The listing builds one solid part. Answer for the finished solid, in the listing's coordinates (mm). A direction names the side the tool comes from. Round coordinates to 2 decimals unless told otherwise and drop trailing zeros. Write each loop counter-clockwise with the first axis right and the second up, starting at its lowest first coordinate (ties: lowest second). Pieces come first, ordered by that corner, then holes.
Item 1: A tool of negligible diameter and unlimited length cuts with its end or side. For faces 1 (the face through (215.9, 19, 627)), 2 (the face through (-4, -3, -609.6)), from which of +Z, -Z, +X, -X, +Y, -Y can it reach the whole face along a straight path? Write none if from no direction.
Item 2: Find the intervals of material crossed by probe 1 along X at (y, z) = (-6, -203); probe 2 along X at (y, z) = (-6, -50); probe 3 along X at (y, z) = (11.5, 946.5), in increasing order.
Item 3: Find section B-B on z = 1362.5. Give the vertices of the cut face in (x, y).
Item 4: Find section A-A on y = 14. Give the vertices of the cut face in (x, z).
Item 5: Find section C-C on x = -20. Give the vertices of the cut face in (y, z).
Item 6: For a pull along X with two mould halves and no side action, classify faces 3 (the face through (-3, 0, 627)), 4 (the face through (304.8, 10, 593)), 5 (the face through (260, 38.1, 627)) as +X half, -X half, draft (parallel to the pull), parting line (faces both ways), or undercut.
```python
from build123d import *

# Parameters (mm, degrees)
F0_W          = 609.6
F0_H          = 1219.2
F1_DEPTH      = 19.05
F2_W          = 88.9
F2_H          = 38.1
F3_DEPTH      = 1219.2
F4_DEPTH      = 2438.4
F4_DEPTH_BACK = 1219.2
F6_R          = 5.55625
F7_DEPTH      = 19.051


with BuildPart() as f1:
    # F0 (on Front) → F1 (new body)
    with BuildSketch(Plane.XZ):
        Rectangle(F0_W, F0_H)
        with Locations((0, 1219.2)):
            Rectangle(F0_W, F0_H)
    extrude(amount=F1_DEPTH)


with BuildPart() as f3:
    # F2 (on face) → F3 (new body)
    with BuildSketch(Plane.XY.offset(1828.8)):
        with Locations((260.35, 19.05)):
            Rectangle(F2_W, F2_H)
        with Locations((-260.35, 19.05)):
            Rectangle(F2_W, F2_H)
    extrude(amount=-F3_DEPTH)


with BuildPart() as f4:
    # F2 (on face) → F4 (new body, two sides)
    with BuildSketch(Plane.XY.offset(1828.8)) as f4_sk:
        with Locations((260.35, 19.05)):
            Rectangle(F2_W, F2_H)
        with Locations((-260.35, 19.05)):
            Rectangle(F2_W, F2_H)
    extrude(amount=-F4_DEPTH)
    extrude(f4_sk.sketch, amount=-F4_DEPTH_BACK)


with BuildPart() as f1_1:
    add(f1.part)

    # F5: union F3, F4
    add(f3.part)
    add(f4.part)

    # F6 (on face) → F7 (cut, through all)
    with BuildSketch(Plane(origin=(0, 0, 0), x_dir=(-1, 0, 0), z_dir=(0, 1, 0))):
        with Locations((-190.5, 1778)):
            Circle(F6_R)
        with Locations((-190.5, 1625.6)):
            Circle(F6_R)
        with Locations((-190.5, 1473.2)):
            Circle(F6_R)
        with Locations((-190.5, 1320.8)):
            Circle(F6_R)
        with Locations((-190.5, 1168.4)):
            Circle(F6_R)
        with Locations((-63.5, 1778)):
            Circle(F6_R)
        with Locations((-63.5, 1625.6)):
            Circle(F6_R)
        with Locations((-63.5, 1473.2)):
            Circle(F6_R)
        with Locations((-63.5, 1320.8)):
            Circle(F6_R)
        with Locations((-63.5, 1168.4)):
            Circle(F6_R)
        with Locations((63.5, 1778)):
            Circle(F6_R)
        with Locations((63.5, 1625.6)):
            Circle(F6_R)
        with Locations((63.5, 1473.2)):
            Circle(F6_R)
        with Locations((63.5, 1320.8)):
            Circle(F6_R)
        with Locations((63.5, 1168.4)):
            Circle(F6_R)
        with Locations((190.5, 1778)):
            Circle(F6_R)
        with Locations((190.5, 1625.6)):
            Circle(F6_R)
        with Locations((190.5, 1473.2)):
            Circle(F6_R)
        with Locations((190.5, 1320.8)):
            Circle(F6_R)
        with Locations((190.5, 1168.4)):
            Circle(F6_R)
        with Locations((-190.5, 1016)):
            Circle(F6_R)
        with Locations((-190.5, 863.6)):
            Circle(F6_R)
        with Locations((-190.5, 711.2)):
            Circle(F6_R)
        with Locations((-190.5, 558.8)):
            Circle(F6_R)
        with Locations((-190.5, 406.4)):
            Circle(F6_R)
        with Locations((-190.5, 254)):
            Circle(F6_R)
        with Locations((-190.5, 101.6)):
            Circle(F6_R)
        with Locations((-190.5, -50.8)):
            Circle(F6_R)
        with Locations((-190.5, -203.2)):
            Circle(F6_R)
        with Locations((-190.5, -355.6)):
            Circle(F6_R)
        with Locations((-63.5, 1016)):
            Circle(F6_R)
        with Locations((-63.5, 863.6)):
            Circle(F6_R)
        with Locations((-63.5, 711.2)):
            Circle(F6_R)
        with Locations((-63.5, 558.8)):
            Circle(F6_R)
        with Locations((-63.5, 406.4)):
            Circle(F6_R)
        with Locations((-63.5, 254)):
            Circle(F6_R)
        with Locations((-63.5, 101.6)):
            Circle(F6_R)
        with Locations((-63.5, -50.8)):
            Circle(F6_R)
        with Locations((-63.5, -203.2)):
            Circle(F6_R)
        with Locations((-63.5, -355.6)):
            Circle(F6_R)
        with Locations((63.5, 1016)):
            Circle(F6_R)
        with Locations((63.5, 863.6)):
            Circle(F6_R)
        with Locations((63.5, 711.2)):
            Circle(F6_R)
        with Locations((63.5, 558.8)):
            Circle(F6_R)
        with Locations((63.5, 406.4)):
            Circle(F6_R)
        with Locations((63.5, 254)):
            Circle(F6_R)
        with Locations((63.5, 101.6)):
            Circle(F6_R)
        with Locations((63.5, -50.8)):
            Circle(F6_R)
        with Locations((63.5, -203.2)):
            Circle(F6_R)
        with Locations((63.5, -355.6)):
            Circle(F6_R)
        with Locations((190.5, 1016)):
            Circle(F6_R)
        with Locations((190.5, 863.6)):
            Circle(F6_R)
        with Locations((190.5, 711.2)):
            Circle(F6_R)
        with Locations((190.5, 558.8)):
            Circle(F6_R)
        with Locations((190.5, 406.4)):
            Circle(F6_R)
        with Locations((190.5, 254)):
            Circle(F6_R)
        with Locations((190.5, 101.6)):
            Circle(F6_R)
        with Locations((190.5, -50.8)):
            Circle(F6_R)
        with Locations((190.5, -203.2)):
            Circle(F6_R)
        with Locations((190.5, -355.6)):
            Circle(F6_R)
        with Locations((-190.5, -508)):
            Circle(F6_R)
        with Locations((-63.5, -508)):
            Circle(F6_R)
        with Locations((63.5, -508)):
            Circle(F6_R)
        with Locations((190.5, -508)):
            Circle(F6_R)
    extrude(amount=-F7_DEPTH, mode=Mode.SUBTRACT)


solid = f1_1.part
```
Check values:
1. face 1: +Z, -Z, +Y
1. face 2: -Z, +X, -X, +Y, -Y
2. probe 1: x = -304.8 to -196.05, -184.95 to -69.05, -57.95 to 57.95, 69.05 to 184.95, 196.05 to 304.8
2. probe 2: x = -304.8 to -196, -185 to -69, -58 to 58, 69 to 185, 196 to 304.8
2. probe 3: x = -304.8 to -215.9, 215.9 to 304.8
3. outline: (-304.8, -19.05) - (304.8, -19.05) - (304.8, 38.1) - (215.9, 38.1) - (215.9, 0) - (-215.9, 0) - (-215.9, 38.1) - (-304.8, 38.1) - close
4. outline: (-304.8, -609.6) - (-215.9, -609.6) - (-215.9, 1828.8) - (-304.8, 1828.8) - close; (215.9, -609.6) - (304.8, -609.6) - (304.8, 1828.8) - (215.9, 1828.8) - close
5. outline: (-19.05, -609.6) - (0, -609.6) - (0, 1828.8) - (-19.05, 1828.8) - close
6. face 3: undercut
6. face 4: +X half
6. face 5: draft
